from build123d import *

# Parameters (mm, degrees)
F0_W     = 1
F0_H     = 35
F1_DEPTH = 2.5


with BuildPart() as f1:
    # F0 (on Top) → F1 (new body, symmetric)
    with BuildSketch(Plane.XY):
        with Locations((-9.75, 18.5)):
            Rectangle(F0_W, F0_H)
        with Locations((9.75, 18.5)):
            Rectangle(F0_W, F0_H)
        Polygon((0, 1), (0, 0), (45.25, 0), (45.25, 1), (10.25, 1), (9.25, 1), align=None)
        Polygon((-45.25, 0), (0, 0), (0, 1), (-9.25, 1), (-10.25, 1), (-45.25, 1), align=None)
    extrude(amount=F1_DEPTH, both=True)


solid = f1.part
The listing builds one solid part. Answer for the finished solid, in the listing's coordinates (mm). A direction names the side the tool comes from. Coordinates: 2 decimals unless noted, no trailing zeros. Loops run counter-clockwise (first coordinate to the right, second up) from the corner with the lowest first, then second, coordinate; pieces in that order, holes last.
1) Determine the mould class of faces 5 (the face through (-10.25, 18, 0)), 6 (the face through (28, 1, 0)), 7 (the face through (0, 1, 0)) for opening direction X: pulls with the +X half, pulls with the -X half, needs draft (parallel to the pull), parting line crosses it, or undercut.
2) Find section B-B on z = -1.3. Write down the section's boundary in (x, y), then the cut area to 4 significant figures.
3) A tool of negligible diameter and unlimited length cuts with its end or side. For faces 1 (the face through (9.25, 18, 0)), 2 (the face through (-28, 1, 0)), 3 (the face through (10, 10, -2.5)), 4 (the face through (10.25, 18, 0)), from which of +Z, -Z, +X, -X, +Y, -Y can it reach the whole face along a straight path? Write none if from no direction.
4) Find section A-A on y = 15. Write down the section's boundary in (x, z), then the cut area to 3 significant figures.
5) Flat-ended cylindrical pins translate along their axes: pin 1 Ø2.5 at (x, z) = (0, -1) entering from +Y; pin 2 Ø1.5 at (y, z) = (20.5, 1) entering from +X. Find the tip coordinate at first contact, or state that the pin passes through.
6) Find section C-C on x = -35. Write down the section's boundary in (y, z), then the cut area to 3 significant figures.
7) Find the intervals of material crossed by L1, parallel to X at y = 13, z = 1; L2, parallel to Y at x = -21.5, z = 1.5, in increasing order.
Values:
1. face 5: pulls with the -X half
1. face 6: needs draft
1. face 7: undercut
2. outline: (-45.25, 0) - (45.25, 0) - (45.25, 1) - (10.25, 1) - (10.25, 36) - (9.25, 36) - (9.25, 1) - (-9.25, 1) - (-9.25, 36) - (-10.25, 36) - (-10.25, 1) - (-45.25, 1) - close
2. area: 160.5 mm2
3. face 1: +Z, -Z, +Y
3. face 2: +Z, -Z, -X, +Y
3. face 3: -Z, +X, -X, +Y, -Y
3. face 4: +Z, -Z, +X, +Y
4. outline: (-10.25, -2.5) - (-9.25, -2.5) - (-9.25, 2.5) - (-10.25, 2.5) - close; (9.25, -2.5) - (10.25, -2.5) - (10.25, 2.5) - (9.25, 2.5) - close
4. area: 10.0 mm2
5. pin 1: stops at y = 1
5. pin 2: stops at x = 10.25
6. outline: (0, -2.5) - (1, -2.5) - (1, 2.5) - (0, 2.5) - close
6. area: 5.00 mm2
7. L1: x = -10.25 to -9.25, 9.25 to 10.25
7. L2: y = 0 to 1
